Geometry: final body of the model. Coordinates: model frame, mm. Give positions to 0.01 mm unless a question says otherwise; leave off trailing zeros. Write each loop counter-clockwise with the first axis right and the second up, starting at its lowest first coordinate (ties: lowest second). Pieces come first, ordered by that corner, then holes. Notation, with made-up numbers: (42, 69) -> (60, 69) arc R16 cw to (60, 85) -> close; hole circle Ø10 at (-3, 14). An arc over 180 degrees is marked (long way). Answer as a JSON object with one key per item and string values. Group by question number.
(1) Contact query for flat-ended pins moving along their axis: pin 1 Ø3 at (x, y) = (-14, 2.5) entering from -Z; pin 2 Ø1.5 at (x, z) = (-12, -2.5) entering from -Y; pin 3 Ø2.5 at (x, y) = (-13.5, 0) entering from +Z. Output: stop coordinate, or through.
(2) Section query D-D on x = -13.5. Output: boundary loops of the cut face in (y, z).
(3) Section query C-C on x = -0.75. Output: boundary loops of the cut face in (y, z).
(4) Section query B-B on z = 0. Output: boundary loops of the cut face in (x, y).
(5) Draft query along Y for faces 1 (the face through (0, -2, 2)), 2 (the face through (-8, -2, 0)), 3 (the face through (-12.96, 0.84, 0.03)). Return one class per face: +Y half, -Y half, draft (parallel to the pull), parting line (faces both ways), or undercut.
(6) Material intervals for probe 1 along X at (y, z) = (0, 0.05); probe 2 along X at (y, z) = (0.5, 0.25); probe 3 along Y at (x, z) = (-13.5, -0.5), sorted ascending.
(7) Section query A-A on y = 0. Output: boundary loops of the cut face in (x, z), plus the area to 3 significant figures.
from build123d import *

# Parameters (mm, degrees)
SKETCH1_R               = 2
BOSS_EXTRUDE1_DEPTH     = 16
SKETCH2_R               = 1
CUT_EXTRUDE1_DEPTH      = 3
CUT_EXTRUDE1_DEPTH_BACK = 3
CHAMFER1_SIZE           = 0.5


with BuildPart() as part:
    # Sketch1 → Boss-Extrude1 (new body)
    with BuildSketch(Plane(origin=(0, 0, 0), x_dir=(0, 0, -1), z_dir=(1, 0, 0))):
        Circle(SKETCH1_R)
    extrude(amount=-BOSS_EXTRUDE1_DEPTH)

    # Sketch2 → Cut-Extrude1 (cut, two sides)
    with BuildSketch(Plane.XY) as cut_extrude1_sk:
        with Locations((-13.5, 0)):
            Circle(SKETCH2_R)
    extrude(amount=CUT_EXTRUDE1_DEPTH, mode=Mode.SUBTRACT)
    extrude(cut_extrude1_sk.sketch, amount=-CUT_EXTRUDE1_DEPTH_BACK, mode=Mode.SUBTRACT)

    # Sketch3 → Revolve1 (revolve)
    with BuildSketch(Plane(origin=(0, 0, 0), x_dir=(1, 0, 0), z_dir=(0, 1, 0))):
        with BuildLine():
            Line((2.757385023, 0), (0, 0))
            Line((0, 0), (0, 3.5))
            ThreePointArc((0, 3.5), (1.985229955, 2.227844932), (2.757385023, 0))
        make_face()
    revolve(axis=Axis((-5.097766842, 0, 0), (1, 0, 0)))

    # Chamfer1
    chamfer1_edges = [part.edges().sort_by_distance(p)[0] for p in [
        (-16, 0, 2),
    ]]
    chamfer(chamfer1_edges, length=CHAMFER1_SIZE)


solid = part.part
Answer list:
{
 "1": {"pin 1": "z = -1.73", "pin 2": "y = -0.97", "pin 3": "z = 2"},
 "2": {"outline": "(-1, -1.73) -> (-1, 1.73) arc R2 ccw to start; (1, -1.73) arc R2 ccw to (1, 1.73) -> close"},
 "3": {"outline": "circle Ø4 at (0, 0)"},
 "4": {"outline": "(-16, -1.5) -> (-15.5, -2) -> (0, -2) -> (0, -3.5) arc R3.6 ccw to (0, 3.5) -> (0, 2) -> (-15.5, 2) -> (-16, 1.5) -> close; hole circle Ø2 at (-13.5, 0)"},
 "5": {"face 1": "draft", "face 2": "parting line", "face 3": "undercut"},
 "6": {"probe 1": "-16 to -14.5, -12.5 to 2.76", "probe 2": "-16 to -14.37, -12.63 to 2.71", "probe 3": "-1.94 to -1, 1 to 1.94"},
 "7": {"outline": "(-16, -1.5) -> (-15.5, -2) -> (-14.5, -2) -> (-14.5, 2) -> (-15.5, 2) -> (-16, 1.5) -> close; (-12.5, -2) -> (0, -2) -> (0, -3.5) arc R3.6 ccw to (0, 3.5) -> (0, 2) -> (-12.5, 2) -> close", "area": "70.1 mm2"}
}
